```python
from build123d import *

# Parameters (mm, degrees)
F0_W     = 203.2
F0_H     = 203.2
F1_DEPTH = 6.35
F2_R     = 6.35
F3_DEPTH = 25.4
F4_R     = 6.35
F5_R     = 38.1
F6_DEPTH = 25.4


with BuildPart() as f1:
    # F0 (on Front) → F1 (new body)
    with BuildSketch(Plane.XZ):
        Rectangle(F0_W, F0_H)
    extrude(amount=F1_DEPTH)

    # F2 (on face) → F3 (cut)
    with BuildSketch(Plane.XZ.offset(6.35)):
        with Locations((-76.2, 76.2)):
            Circle(F2_R)
        with Locations((76.2, 76.2)):
            Circle(F2_R)
        with Locations((-76.2, -76.2)):
            Circle(F2_R)
        with Locations((76.2, -76.2)):
            Circle(F2_R)
    extrude(amount=-F3_DEPTH, mode=Mode.SUBTRACT)

    # F4
    f4_edges = [f1.edges().sort_by_distance(p)[0] for p in [
        (101.6, -3.175, 101.6),
        (-101.6, -3.175, 101.6),
        (-101.6, -3.175, -101.6),
        (101.6, -3.175, -101.6),
    ]]
    fillet(f4_edges, radius=F4_R)

    # F5 (on face) → F6 (cut)
    with BuildSketch(Plane.XZ.offset(6.35)):
        with Locations((50.8, 25.4)):
            Circle(F5_R)
    extrude(amount=-F6_DEPTH, mode=Mode.SUBTRACT)


solid = f1.part
```
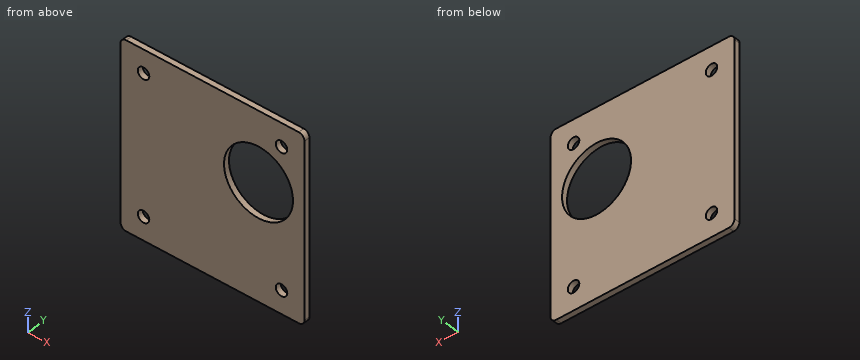
CAD build for the part. Positions are in the model's coordinates, mm. Give positions to 0.01 mm unless a question says otherwise; leave off trailing zeros. Loops run counter-clockwise (first coordinate to the right, second up) from the corner with the lowest first, then second, coordinate; pieces in that order, holes last. Notation, with made-up numbers: M -25.75,53 L -7.75,53 A13 ccw -7.75,76 Z; hole C 62,-16 d11. An arc over 180 degrees is marked long. Use one line per item in the form item = value.
Item 1: Slice it at B-B (x = 50.8). List the corners of the cut face in (y, z), plus the area to 3 significant figures.
Determined:
outline = M -6.35,-101.6 L 0,-101.6 L 0,-12.7 L -6.35,-12.7 Z; M -6.35,63.5 L 0,63.5 L 0,101.6 L -6.35,101.6 Z
area = 806 mm2
Item 2: Slice it at D-D (z = 76.2). List the corners of the cut face in (x, y).
Determined:
outline = M -101.6,-6.35 L -82.55,-6.35 L -82.55,0 L -101.6,0 Z; M -69.85,-6.35 L 69.85,-6.35 L 69.85,0 L -69.85,0 Z; M 82.55,-6.35 L 101.6,-6.35 L 101.6,0 L 82.55,0 Z
Item 3: Flat gauge pins, fed straight in: pin 1 (20.5 mm diameter, centred on x = 76.2, z = -76.2, fed in from -Y); pin 2 (7.5 mm diameter, centred on x = 76.2, z = 76.2, fed in from -Y). Where does each tip first touch, or does it go through?
Determined:
pin_1 = -6.35
pin_2 = through
Item 4: Slice it at A-A (z = 25.4). List the corners of the cut face in (x, y), plus the area to 3 significant figures.
Determined:
outline = M -101.6,-6.35 L 12.7,-6.35 L 12.7,0 L -101.6,0 Z; M 88.9,-6.35 L 101.6,-6.35 L 101.6,0 L 88.9,0 Z
area = 806 mm2
Item 5: Slice it at C-C (y = -2.5). List the corners of the cut face in (x, z).
Determined:
outline = M -101.6,-95.25 A6.35 ccw -95.25,-101.6 L 95.25,-101.6 A6.35 ccw 101.6,-95.25 L 101.6,95.25 A6.35 ccw 95.25,101.6 L -95.25,101.6 A6.35 ccw -101.6,95.25 Z; hole C -76.2,-76.2 d12.7; hole C -76.2,76.2 d12.7; hole C 50.8,25.4 d76.2; hole C 76.2,-76.2 d12.7; hole C 76.2,76.2 d12.7
Item 6: Drill centre lines: probe 1 along Z at (x, y) = (76.2, -1.25); probe 2 along Z at (x, y) = (50.8, -3.25); probe 3 along Z at (x, y) = (76, -1). Where is each one in solid material? Low to high. Write a range as from..to.
Determined:
probe_1 = -101.6..-82.55, -69.85..-3, 53.8..69.85, 82.55..101.6
probe_2 = -101.6..-12.7, 63.5..101.6
probe_3 = -101.6..-82.55, -69.85..-3.18, 53.98..69.85, 82.55..101.6
